Could you check a few things on this drawing? It's one solid part, dimensions in mm from its lowest x, y, z. Give positions to 0.01 mm unless a question says otherwise; leave off trailing zeros. Order: outer loops, then holes, each group sorted by start corner. A loop starts at its lowest first (then second) coordinate and runs counter-clockwise, first axis right, second up.
Item 1: I'm going to push flat-ended pins straight in: pin 1 Ø5 at (x, z) = (28.5, 53.25) entering from -Y; pin 2 Ø3 at (y, z) = (106, 31) entering from +X; pin 3 Ø1 at (y, z) = (40.5, 33) entering from -X; pin 4 Ø4 at (x, z) = (3.75, 28.5) entering from -Y. Where does each tip first touch, or does it pass through?
Item 2: If we mould it in two halves opening along Z, with no side actions, what happens to the marked faces 1, 2 and 3? For each: +Z half, -Z half, draft (parallel to the pull), parting line (faces both ways), or undercut.
Item 3: If I drill on line 1 along Z through (x, y) = (28, 82); line 2 along X through (y, z) = (1, 28), over which ranges is the centre line in solid material (lowest first)?
Item 4: I want a section at C-C, the plane x = 10.5. Write out the boundary of the cut face in (y, z).
Item 5: I want a section at D-D, the plane z = 47. Write out the boundary of the cut face in (x, y).
Item 6: I want a section at A-A, the plane z = 28.5. Write out the boundary of the cut face in (x, y), then the cut area to 3 significant figures.
Item 7: I want a section at B-B, the plane y = 115.35. Write out the boundary of the cut face in (x, z).
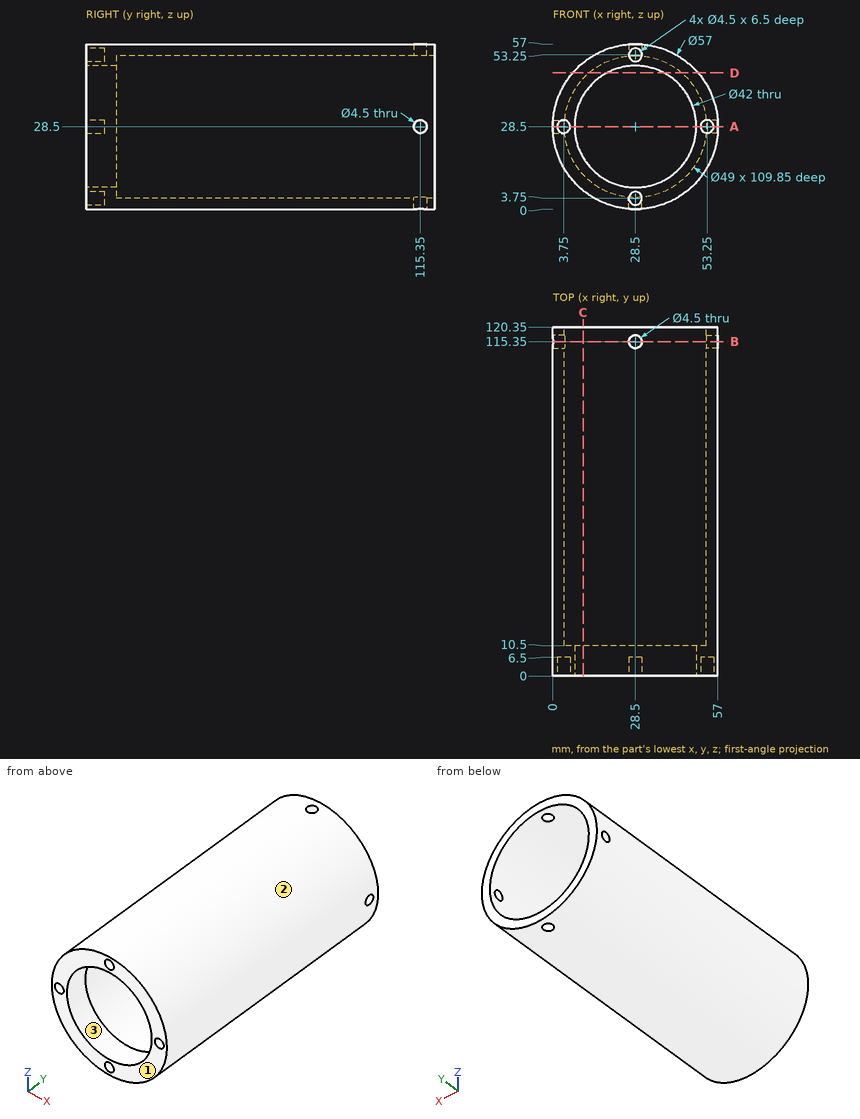
Results list:
1. pin 1: stops at y = 0
1. pin 2: stops at x = 56.98
1. pin 3: stops at x = 0.28
1. pin 4: stops at y = 6.5
2. face 1: draft
2. face 2: parting line
2. face 3: undercut
3. line 1: z = 0 to 4.01, 52.99 to 57
3. line 2: x = 0 to 1.56, 5.94 to 7.51, 49.49 to 51.06, 55.44 to 57
4. outline: (0, 6.4) - (120.35, 6.4) - (120.35, 11.88) - (10.5, 11.88) - (10.5, 17.68) - (0, 17.68) - close; (0, 39.32) - (10.5, 39.32) - (10.5, 45.12) - (120.35, 45.12) - (120.35, 50.6) - (0, 50.6) - close
5. outline: (6.82, 0) - (18.56, 0) - (18.56, 10.5) - (12.44, 10.5) - (12.44, 120.35) - (6.82, 120.35) - close; (38.44, 0) - (50.18, 0) - (50.18, 120.35) - (44.56, 120.35) - (44.56, 10.5) - (38.44, 10.5) - close
6. outline: (0, 0) - (1.5, 0) - (1.5, 6.5) - (6, 6.5) - (6, 0) - (7.5, 0) - (7.5, 10.5) - (4, 10.5) - (4, 113.1) - (0, 113.1) - close; (0, 117.6) - (4, 117.6) - (4, 120.35) - (0, 120.35) - close; (49.5, 0) - (51, 0) - (51, 6.5) - (55.5, 6.5) - (55.5, 0) - (57, 0) - (57, 113.1) - (53, 113.1) - (53, 10.5) - (49.5, 10.5) - close; (53, 117.6) - (57, 117.6) - (57, 120.35) - (53, 120.35) - close
6. area: 942 mm2
7. outline: (0.09, 26.25) arc R28.5 ccw to (26.25, 0.09) - (26.25, 4.1) arc R24.5 cw to (4.1, 26.25) - close; (0.09, 30.75) - (4.1, 30.75) arc R24.5 cw to (26.25, 52.9) - (26.25, 56.91) arc R28.5 ccw to start; (30.75, 0.09) arc R28.5 ccw to (56.91, 26.25) - (52.9, 26.25) arc R24.5 cw to (30.75, 4.1) - close; (30.75, 52.9) arc R24.5 cw to (52.9, 30.75) - (56.91, 30.75) arc R28.5 ccw to (30.75, 56.91) - close
